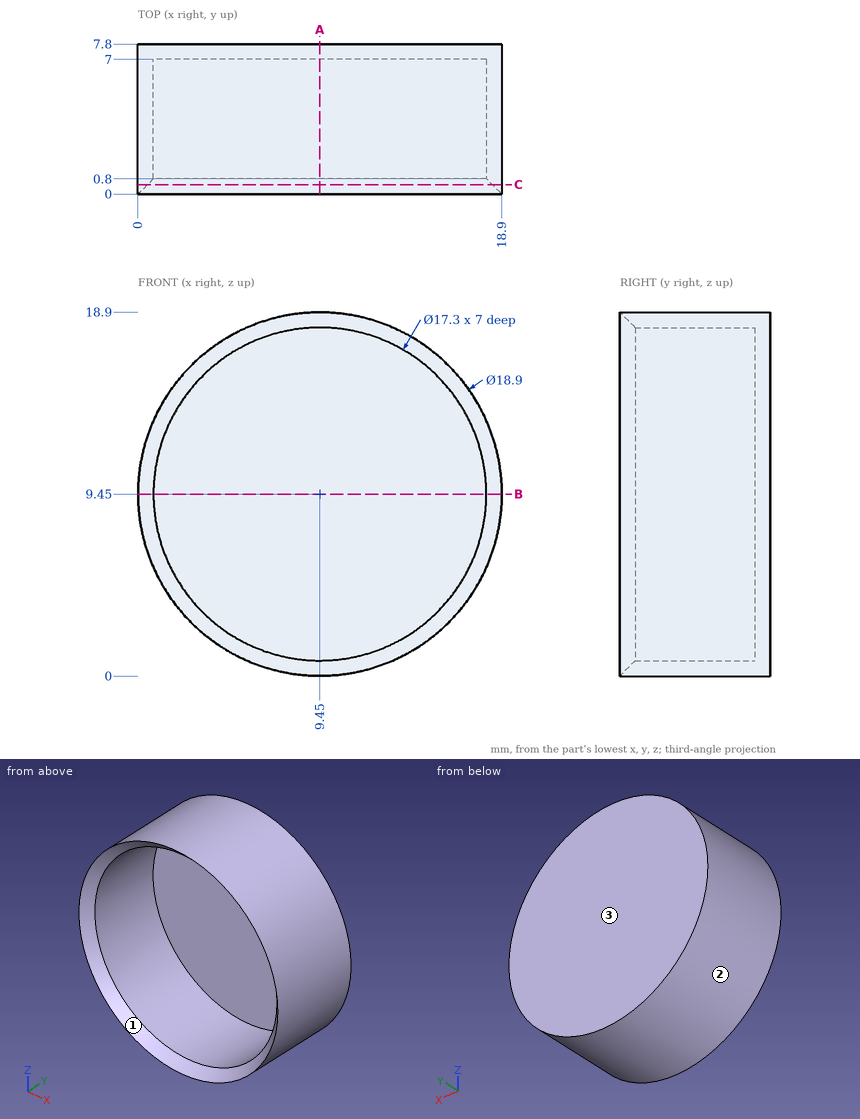
Can you work these out from the drawing? Everything is in mm from the part's minimum corner. Give positions to 0.01 mm unless a question says otherwise; leave off trailing zeros. Write each loop counter-clockwise with the first axis right and the second up, starting at its lowest first coordinate (ties: lowest second). Pieces come first, ordered by that corner, then holes. Notation, with made-up numbers: (-39, 60) -> (-24, 60) arc R13 cw to (-24, 75) -> close; hole circle Ø2 at (-7.5, 58.25). An arc over 180 degrees is marked (long way). Write each question's results on one line, items separated by ' | '.
Item 1: For pin 1 Ø8 at (x, z) = (13, 11.5) entering from -Y; pin 2 Ø1 at (x, y) = (10.5, 5) entering from +Z; pin 3 Ø1.5 at (x, z) = (16, 4.5) entering from -Y, each with a flat end and sliding along its axis, tell me the tip position at first contact or that it passes through.
Output:
pin 1: stops at y = 7 | pin 2: stops at z = 18.88 | pin 3: stops at y = 0.49
Item 2: We'd pull the mould along X, two halves only. Please class the marked faces 1, 2 and 3: pulls with the +X half, pulls with the -X half, needs draft (parallel to the pull), parting line crosses it, or undercut.
Output:
face 1: undercut | face 2: parting line crosses it | face 3: needs draft
Item 3: Suppose I cut it at C-C on y = 0.5. Write out the boundary of the cut face in (x, z).
Output:
outline: circle Ø18.9 at (9.45, 9.45); hole circle Ø17.9 at (9.45, 9.45)
Item 4: If I drill on L1, parallel to Z at x = 9.45, y = 3.25; L2, parallel to Y at x = 17.25, z = 9.75; L3, parallel to Z at x = 7.25, y = 6.25, over which ranges is the centre line in solid material (lowest first)?
Output:
L1: z = 0 to 0.8, 18.1 to 18.9 | L2: y = 7 to 7.8 | L3: z = 0.26 to 1.08, 17.82 to 18.64
Item 5: Suppose I cut it at A-A on x = 9.45. Write out the boundary of the cut face in (y, z), plus the area to 3 significant figures.
Output:
outline: (0, 0) -> (7.8, 0) -> (7.8, 18.9) -> (0, 18.9) -> (0.8, 18.1) -> (7, 18.1) -> (7, 0.8) -> (0.8, 0.8) -> close | area: 25.7 mm^2
Item 6: Suppose I cut it at B-B on z = 9.45. Write out the boundary of the cut face in (x, y).
Output:
outline: (0, 0) -> (0.8, 0.8) -> (0.8, 7) -> (18.1, 7) -> (18.1, 0.8) -> (18.9, 0) -> (18.9, 7.8) -> (0, 7.8) -> close
